Input: part model. Units: mm. Frame: model coordinates. A direction names the side the tool comes from. Coordinates: 2 decimals unless noted, no trailing zeros. Loops run counter-clockwise (first coordinate to the right, second up) from the corner with the lowest first, then second, coordinate; pieces in that order, holes last.
Item 1: Section C-C on z = 0. Return loops of the section in (x, y).
Item 2: Contact query for flat-ended pins moving along their axis: P1, Ø5, axis at x = 40, z = 24.5, coming from the -Y side; P2, Ø10, axis at x = -17.5, z = -1.5, coming from the +Y side. Output: stop coordinate, or through.
Item 3: Pull-direction query (Z, two-part tool) for faces 1 (the flat face through (59, -3, -1)), 2 (the flat face through (-60, -3, -1)), 3 (the flat face through (-1, -3, 43)); classes: released by +Z, released by -Z, zero draft, split by the parting line, or undercut.
Item 4: Section B-B on x = -30.25. Return loops of the section in (y, z).
Item 5: Reachability of faces 4 (the flat face through (-1, -3, -42)), 5 (the flat face through (60, -3, -1)) from +Z, -Z, +X, -X, +Y, -Y: full face, straight path, thin tool, end or side. Return the list, or none.
Item 6: Section D-D on z = 15.5. Return loops of the section in (x, y).
Item 7: Ray query, line 1 along Z through (x, y) = (20, -1.6); line 2 along X through (y, z) = (-5.05, 11); line 3 along Y through (x, z) = (-33, -14.5). Return the intervals inside material, ascending.
Item 8: Section A-A on z = -9. Return loops of the section in (x, y).
```python
from build123d import *

# Parameters (mm, degrees)
F0_W     = 120
F0_H     = 86
F0_W_2   = 20
F0_H_2   = 14
F1_DEPTH = 6
F2_R     = 2
F3_T     = -1


with BuildPart() as f1:
    # F0 (on Front) → F1 (new body)
    with BuildSketch(Plane.XZ):
        Rectangle(F0_W, F0_H)
        with Locations((0, -5)):
            Rectangle(F0_W_2, F0_H_2, mode=Mode.SUBTRACT)
        with BuildLine():
            Line((-28.5, 4.5), (-28.5, -4.5))
            ThreePointArc((-28.5, -4.5), (-30.25, -6.25), (-32, -4.5))
            Line((-32, -4.5), (-32, 4.5))
            ThreePointArc((-32, 4.5), (-30.25, 6.25), (-28.5, 4.5))
        make_face(mode=Mode.SUBTRACT)
        with BuildLine():
            Line((34.75, -1.75), (25.75, -1.75))
            ThreePointArc((25.75, -1.75), (24, 0), (25.75, 1.75))
            Line((25.75, 1.75), (34.75, 1.75))
            ThreePointArc((34.75, 1.75), (36.5, 0), (34.75, -1.75))
        make_face(mode=Mode.SUBTRACT)
    extrude(amount=F1_DEPTH)

    # F2
    f2_edges = [f1.edges().sort_by_distance(p)[0] for p in [
        (-60, -3, -43),
        (-60, -3, 43),
        (60, -3, 43),
        (60, -3, -43),
    ]]
    fillet(f2_edges, radius=F2_R)

    # F3
    f3_openings = [f1.faces().sort_by_distance(p)[0] for p in [
        (-28.5, -3, 0),
        (-30.25, -3, 6.25),
        (-32, -3, 0),
        (-30.25, -3, -6.25),
        (10, -3, -5),
        (0, -3, 2),
        (58.523653, -6, 0),
        (0, -3, -12),
        (-10, -3, -5),
        (30.25, -3, 1.75),
        (36.5, -3, 0),
        (24, -3, 0),
        (30.25, -3, -1.75),
    ]]
    offset(amount=F3_T, openings=f3_openings)


solid = f1.part
```
Results found:
1. outline: (-60, -6) - (-59, -6) - (-59, -1) - (-32, -1) - (-32, 0) - (-60, 0) - close; (-28.5, -1) - (-10, -1) - (-10, 0) - (-28.5, 0) - close; (10, -1) - (24, -1) - (24, 0) - (10, 0) - close; (36.5, -1) - (59, -1) - (59, -6) - (60, -6) - (60, 0) - (36.5, 0) - close
2. P1: stops at y = -1
2. P2: stops at y = 0
3. face 1: undercut
3. face 2: zero draft
3. face 3: released by +Z
4. outline: (-6, -43) - (0, -43) - (0, -6.25) - (-1, -6.25) - (-1, -42) - (-6, -42) - close; (-6, 42) - (-1, 42) - (-1, 6.25) - (0, 6.25) - (0, 43) - (-6, 43) - close
5. face 4: -Y
5. face 5: +Z, -Z, +X, +Y, -Y
6. outline: (-60, -6) - (-59, -6) - (-59, -1) - (59, -1) - (59, -6) - (60, -6) - (60, 0) - (-60, 0) - close
7. line 1: z = -43 to -42, 42 to 43
7. line 2: x = -60 to -59, 59 to 60
7. line 3: y = -1 to 0
8. outline: (-60, -6) - (-59, -6) - (-59, -1) - (-10, -1) - (-10, 0) - (-60, 0) - close; (10, -1) - (59, -1) - (59, -6) - (60, -6) - (60, 0) - (10, 0) - close
